Here's how the part is built. I have some questions about the finished solid (model axes, mm). A direction names the side the tool comes from. Round coordinates to 2 decimals unless told otherwise and drop trailing zeros. Loops run counter-clockwise (first coordinate to the right, second up) from the corner with the lowest first, then second, coordinate; pieces in that order, holes last. Notation, with made-up numbers: M 66.25,65.5 L 80.25,65.5 A13 cw 80.25,78.5 Z; hole C 75,11 d8. An arc over 180 degrees is marked long. Answer as CSV lines item,"result".
```python
from build123d import *

# Parameters (mm, degrees)
BASE_FLANGE1_DEPTH           = 306.832
SKETCH2_W                    = 2.032
SKETCH2_H                    = 34.036
BOSS_EXTRUDE1_DEPTH          = 25.4
EDGE_FLANGE1_STRIP_W         = 14.478
EDGE_FLANGE1_STRIP_H         = 2.032
EDGE_FLANGE1_STRIP_CUT_DEPTH = 34.036
EDGE_FLANGE1_DEPTH           = 34.036
SKETCH6_R                    = 2.4511
CUT_EXTRUDE1_DEPTH           = 338.350728951
SKETCH7_R                    = 4.3688
CUT_EXTRUDE2_DEPTH           = 338.350728951
SKETCH8_R                    = 2.4511
CUT_EXTRUDE3_DEPTH           = 363.392135571
FILLET1_R                    = 3.175


# Sheet-metal steps are written as plain solids
with BuildPart() as part:
    # Sketch1 → Base-Flange1 (new body)
    with BuildSketch(Plane(origin=(0, 0, 0), x_dir=(0, 0, -1), z_dir=(1, 0, 0))):
        with BuildLine():
            Line((22.225, 0), (5.207, 0))
            ThreePointArc((5.207, 0), (1.52509499, 1.52509499), (0, 5.207))
            Line((0, 5.207), (0, 39.243))
            ThreePointArc((0, 39.243), (1.52509499, 42.92490501), (5.207, 44.45))
            Line((5.207, 44.45), (22.225, 44.45))
            Line((22.225, 44.45), (22.225, 42.418))
            Line((22.225, 42.418), (5.207, 42.418))
            ThreePointArc((5.207, 42.418), (2.96193597, 41.48806403), (2.032, 39.243))
            Line((2.032, 39.243), (2.032, 5.207))
            ThreePointArc((2.032, 5.207), (2.96193597, 2.96193597), (5.207, 2.032))
            Line((5.207, 2.032), (22.225, 2.032))
            Line((22.225, 2.032), (22.225, 0))
        make_face()
    extrude(amount=BASE_FLANGE1_DEPTH)

    # Sketch2 → Boss-Extrude1 (add)
    with BuildSketch(Plane(origin=(306.832, 0, 0), x_dir=(0, 0, -1), z_dir=(1, 0, 0))):
        with Locations((1.016, 22.225)):
            Rectangle(SKETCH2_W, SKETCH2_H)
    boss_extrude1 = extrude(amount=BOSS_EXTRUDE1_DEPTH)

    # Edge-Flange1 strip (across the edge) → Edge-Flange1 strip cut (cut)
    with BuildSketch(Plane(origin=(332.232, 39.243, -2.032), x_dir=(-1, 0, 0), z_dir=(0, -1, 0))):
        with Locations((-2.032, -1.016)):
            Rectangle(EDGE_FLANGE1_STRIP_W, EDGE_FLANGE1_STRIP_H)
    edge_flange1_strip_cut = extrude(amount=EDGE_FLANGE1_STRIP_CUT_DEPTH, mode=Mode.SUBTRACT)

    # Edge-Flange1 section (across the edge) → Edge-Flange1 (add)
    with BuildSketch(Plane(origin=(332.232, 39.243, -2.032), x_dir=(-1, 0, 0), z_dir=(0, -1, 0))):
        with BuildLine():
            Line((0, 3.175), (0, 36.068))
            Line((0, 36.068), (2.032, 36.068))
            Line((2.032, 36.068), (2.032, 3.175))
            ThreePointArc((2.032, 3.175), (2.96193597, 0.92993597), (5.207, 0))
            Line((5.207, 0), (5.207, -2.032))
            ThreePointArc((5.207, -2.032), (1.52509499, -0.50690501), (0, 3.175))
        make_face()
    edge_flange1 = extrude(amount=EDGE_FLANGE1_DEPTH)

    # Mirror1: Boss-Extrude1, Edge-Flange1 strip cut, Edge-Flange1 across plane
    add(boss_extrude1.mirror(Plane.ZY.offset(-153.416)))
    add(edge_flange1_strip_cut.mirror(Plane.ZY.offset(-153.416)), mode=Mode.SUBTRACT)
    add(edge_flange1.mirror(Plane.ZY.offset(-153.416)))

    # Sketch6 → Cut-Extrude1 (cut, through all)
    with BuildSketch(Plane(origin=(0, 44.45, 0), x_dir=(1, 0, 0), z_dir=(0, 1, 0))):
        with Locations(Location((25.4, 15.875, 0), (0, 0, 270))):
            Circle(SKETCH6_R)
        with Locations(Location((281.432, 15.875, 0), (0, 0, 270))):
            Circle(SKETCH6_R)
    extrude(amount=-CUT_EXTRUDE1_DEPTH, mode=Mode.SUBTRACT)

    # Sketch7 → Cut-Extrude2 (cut, through all)
    with BuildSketch(Plane.XY):
        with Locations((0, 22.225)):
            Circle(SKETCH7_R)
        with Locations((306.832, 22.225)):
            Circle(SKETCH7_R)
    extrude(amount=-CUT_EXTRUDE2_DEPTH, mode=Mode.SUBTRACT)

    # Sketch8 → Cut-Extrude3 (cut, through all)
    with BuildSketch(Plane(origin=(332.232, 0, 0), x_dir=(0, 0, -1), z_dir=(1, 0, 0))):
        with Locations((31.75, 22.225)):
            Circle(SKETCH8_R)
        with Locations((12.7, 22.225)):
            Circle(SKETCH8_R)
    extrude(amount=-CUT_EXTRUDE3_DEPTH, mode=Mode.SUBTRACT)

    # Fillet1
    fillet1_edges = [part.edges().sort_by_distance(p)[0] for p in [
        (-24.384, 5.207, -38.1),
        (0, 1.016, -22.225),
        (-24.384, 39.243, -38.1),
        (0, 43.434, -22.225),
        (306.832, 1.016, -22.225),
        (331.216, 39.243, -38.1),
        (331.216, 5.207, -38.1),
        (306.832, 43.434, -22.225),
    ]]
    fillet(fillet1_edges, radius=FILLET1_R)


solid = part.part
```
1. For P1, Ø18.5, axis at x = 198, z = -17, coming from the -Y side; P2, Ø3, axis at x = 25.4, z = -15.875, coming from the -Y side; P3, Ø8, axis at x = 53.5, y = 26.5, coming from the -Z side, each with a flat end and sliding along its axis, tell me the tip position at first contact or that it passes through.
Evaluation:
P1,"stops at y = 0"
P2,"passes through"
P3,"stops at z = -2.03"
2. Which directions (+Z, -Z, +X, -X, +Y, -Y) give clear straight access to the entire face, cutting with the end or side of a thin tool? Please do faces 5 (the flat face through (330.2, 22, -22)), 6 (the flat face through (156, 22, -2.032)), 7 (the flat face through (-24, 5.207, -10)), 8 (the flat face through (151, 42.418, -14)).
Evaluation:
face 5,"-Z, +Y, -Y"
face 6,"-Z"
face 7,"+Z, -Z, -X, -Y"
face 8,"-Z, +X, -X"
3. I want a section at A-A, the plane x = 71.5. Please give me the cut outline in (y, z) (3 decimals).
Evaluation:
outline,"M 0,-22.225 L 2.032,-22.225 L 2.032,-5.207 A3.175 cw 5.207,-2.032 L 39.243,-2.032 A3.175 cw 42.418,-5.207 L 42.418,-22.225 L 44.45,-22.225 L 44.45,-5.207 A5.207 ccw 39.243,0 L 5.207,0 A5.207 ccw 0,-5.207 Z"
4. If I drill on line 1 (X direction, y = 29.5, z = -35); line 2 (Y direction, x = 125.5, z = -22); line 3 (Y direction, x = 331.5, z = -12.7), over which ranges is the centre line in solid material (lowest first)? Write a range as [from, to].
Evaluation:
line 1,"x = [-25.4, -23.37], [330.2, 332.23]"
line 2,"y = [0, 2.03], [42.42, 44.45]"
line 3,"y = [5.21, 19.77], [24.68, 39.24]"
5. I want a section at B-B, the plane y = 13.5. Please give me the cut outline in (x, z) (3 decimals), and give its area (3 significant figures).
Evaluation:
outline,"M -25.4,-38.1 L -23.368,-38.1 L -23.368,-5.207 A3.175 cw -20.193,-2.032 L 327.025,-2.032 A3.175 cw 330.2,-5.207 L 330.2,-38.1 L 332.232,-38.1 L 332.232,-5.207 A5.207 ccw 327.025,0 L -20.193,0 A5.207 ccw -25.4,-5.207 Z"
area,"866 mm²"
6. We'd pull the mould along Y, two halves only. Please class faces 1 (the cylindrical face through (-3.2, 25.2, -1)), 2 (the flat face through (-23.368, 22, -22)), 3 (the cylindrical face through (303.612, 25.178, -1.002)), 4 (the flat face through (-24, 39.243, -10)): pulls with the +Y half, pulls with the -Y half, needs draft (parallel to the pull), parting line crosses it, or undercut.
Evaluation:
face 1,"undercut"
face 2,"needs draft"
face 3,"undercut"
face 4,"pulls with the +Y half"
